Could you check a few things on this model? Use its own coordinates, in mm. Face numbers are marked on the shaded views. A direction names the side the tool comes from. Give positions to 0.01 mm unless a question says otherwise; leave off trailing zeros. Order: outer loops, then holes, each group sorted by start corner. A loop starts at its lowest first (then second) coordinate and runs counter-clockwise, first axis right, second up. Notation, with made-up numbers: (-4, 25) -> (55, 25) arc R38 cw to (55, 64) -> close; hole circle Ø6 at (37, 60). An arc over 180 degrees is marked (long way). Answer as CSV lines item,"result". Start each with the question number.
(1) We'd pull the mould along Z, two halves only. Please class the marked faces 1, 2 and 3: released by +Z, released by -Z, zero draft, split by the parting line, or undercut.
(2) On a 3-axis mill with a long thin cutter (end or side, diameter ignored), from which of +Z, -Z, +X, -X, +Y, -Y can I reach the whole of each face in a straight line? I mean the marked faces 4 and 5. Say none if no direction works.
(3) I want a section at C-C (x = -2.7). Please give me the cut outline in (y, z).
(4) Will these pins go through, and if not, where does the flat tip stop? pin 1 Ø2 at (x, y) = (-4, 0) entering from +Z; pin 2 Ø1 at (x, y) = (-1.5, -1.5) entering from -Z; pin 3 Ø1 at (x, y) = (-3.5, -2) entering from +Z.
(5) I need wall thicknesses on L1, parallel to Z at x = -3.1, y = 0; L2, parallel to X at y = 1.8, z = -1.5; L3, parallel to Z at x = -1.5, y = -0.8. Which ranges of each line are inside material? Lowest first, please.
(6) I want a section at A-A (z = 0). Please give me the cut outline in (x, y).
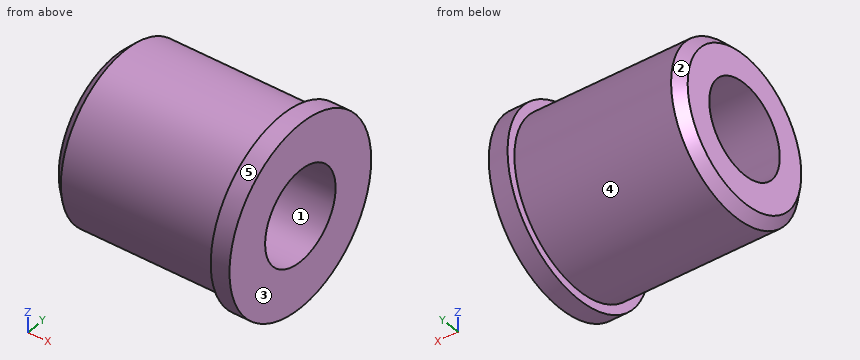
```python
from build123d import *

# Parameters (mm, degrees)
M3X0_25_4H_TAPPED_HOLE1_D = 2.4892


with BuildPart() as part:
    # Sketch1 one side → Revolve1 (revolve)
    with BuildSketch(Plane.XY, mode=Mode.PRIVATE) as revolve1_sk:
        Polygon((-0.508, -2.5019), (0, -2.5019), (0, 0), (-5.0038, 0), (-5.0038, -2.0066), (-4.7498, -2.2606), (-0.508, -2.2606), align=None)
    revolve(revolve1_sk.sketch.rotate(Axis((0, 0, 0), (-1, 0, 0)), 180), axis=Axis((0, 0, 0), (-1, 0, 0)))  # turned: the seam where the file's is

    # M3x0.25-4h Tapped Hole1 (through all)
    with Locations(Plane.YZ):
        with Locations((0, 0)):
            Hole(M3X0_25_4H_TAPPED_HOLE1_D / 2)


solid = part.part
```
Final values:
1,face 1,"undercut"
1,face 2,"split by the parting line"
1,face 3,"zero draft"
2,face 4,"-X"
2,face 5,"+X, -X"
3,outline,"circle Ø4.52 at (0, 0); hole circle Ø2.49 at (0, 0)"
4,pin 1,"z = 2.26"
4,pin 2,"z = -2.03"
4,pin 3,"z = 1.69"
5,L1,"-2.26 to -1.24, 1.24 to 2.26"
5,L2,"-0.51 to 0"
5,L3,"-2.11 to -0.95, 0.95 to 2.11"
6,outline,"(-5, -2.01) -> (-4.75, -2.26) -> (-0.51, -2.26) -> (-0.51, -2.5) -> (0, -2.5) -> (0, -1.24) -> (-5, -1.24) -> close; (-5, 1.24) -> (0, 1.24) -> (0, 2.5) -> (-0.51, 2.5) -> (-0.51, 2.26) -> (-4.75, 2.26) -> (-5, 2.01) -> close"
